```python
from build123d import *

# Parameters (mm, degrees)
F0_W      = 300
F0_H      = 10
F1_DEPTH  = 300
F2_W      = 25
F2_H      = 25
F3_DEPTH  = 10
F4_W      = 20
F4_H      = 10
F5_DEPTH  = 1
F6_W      = 20
F6_H      = 10
F7_DEPTH  = 1
F8_W      = 1
F8_H      = 20
F9_DEPTH  = 200
F10_W     = 300
F10_H     = 10
F11_DEPTH = 300


with BuildPart() as f1:
    # F0 (on Front) → F1 (new body)
    with BuildSketch(Plane.XZ):
        with Locations((102.931539, 34.842865)):
            Rectangle(F0_W, F0_H)
    extrude(amount=F1_DEPTH)

    # F2 (on face) → F3 (join)
    with BuildSketch(Plane(origin=(0, 0, 29.842865), x_dir=(1, 0, 0), z_dir=(0, 0, -1))):
        with Locations((240.431539, 12.5)):
            Rectangle(F2_W, F2_H)
        with Locations((-34.568461, 12.5)):
            Rectangle(F2_W, F2_H)
        with Locations((240.431539, 287.5)):
            Rectangle(F2_W, F2_H)
        with Locations((-34.568461, 287.5)):
            Rectangle(F2_W, F2_H)
    extrude(amount=F3_DEPTH)

    # F4 (on face) → F5 (join)
    with BuildSketch(Plane.YZ.offset(252.931539)):
        with Locations((-45, 34.842865)):
            Rectangle(F4_W, F4_H)
        with Locations((-255, 34.842865)):
            Rectangle(F4_W, F4_H)
    extrude(amount=F5_DEPTH)

    # F6 (on face) → F7 (join)
    with BuildSketch(Plane(origin=(-47.068461, 0, 0), x_dir=(0, -1, 0), z_dir=(-1, 0, 0))):
        with Locations((45, 34.842865)):
            Rectangle(F6_W, F6_H)
        with Locations((255, 34.842865)):
            Rectangle(F6_W, F6_H)
    extrude(amount=F7_DEPTH)

    # F8 (on face) → F9 (join)
    with BuildSketch(Plane.XY.offset(39.842865)):
        with Locations((253.431539, -45)):
            Rectangle(F8_W, F8_H)
        with Locations((253.431539, -255)):
            Rectangle(F8_W, F8_H)
        with Locations((-47.568461, -255)):
            Rectangle(F8_W, F8_H)
        with Locations((-47.568461, -45)):
            Rectangle(F8_W, F8_H)
    extrude(amount=F9_DEPTH)

    # F10 (on face) → F11 (join)
    with BuildSketch(Plane(origin=(252.931539, 0, 0), x_dir=(0, -1, 0), z_dir=(-1, 0, 0))):
        with Locations((150, 234.842865)):
            Rectangle(F10_W, F10_H)
    extrude(amount=F11_DEPTH)


solid = f1.part
```
Check sheet for the modelled part. Datum: model origin and axes. Units: mm. A direction names the side the tool comes from. Give positions to 0.01 mm unless a question says otherwise; leave off trailing zeros. Write each loop counter-clockwise with the first axis right and the second up, starting at its lowest first coordinate (ties: lowest second). Pieces come first, ordered by that corner, then holes. Notation, with made-up numbers: (-22, 65) -> (27, 65) arc R36 ccw to (27, 102) -> close; hole circle Ø6 at (1, 1.5). An arc over 180 degrees is marked (long way). Use CSV: the item, a comma, the result in double quotes. Start each with the question number.
Q1. Scan lines: line 1 along Z through (x, y) = (110, -73); line 2 along X through (y, z) = (-258.5, 58.5). Record each from-to range of solid material in increasing order.
Q2. Cross-section at B-B on y = -61. Enter the section's corners in (x, z).
Q3. Cross-section at C-C on x = 177. Enter the section's corners in (y, z), and give its area (3 significant figures).
Q4. Release check for a two-part mould opening along Y. For faces 6 (the flat face through (105, -148, 239.843)), 7 (the flat face through (240, -25, 25)), 8 (the flat face through (105, 0, 235)) record: +Y half, -Y half, draft (parallel to the pull), parting line (faces both ways), or undercut.
Q5. Tool access check on faces 1 (the flat face through (-47.068, -149, 235)), 2 (the flat face through (-22.068, -12, 25)), 3 (the flat face through (252.932, -255, 134)), 4 (the flat face through (252.932, -17, 235)), 5 (the flat face through (-47.068, -286, 30)). Record the directions out of +Z, -Z, +X, -X, +Y, -Y that give a thin tool (end or side, any length) a straight path to the whole face; none if there is none.
Q6. Depth check by flat-ended pin: P1, Ø10, axis at y = -275, z = 25, coming from the -X side; P2, Ø3, axis at y = -26, z = 235.5, coming from the +X side; P3, Ø1.1, axis at x = 253.5, z = 178, coming from the -Y side. Enter the tip coordinate at first touch or a pass-through.
Q7. Cross-section at A-A on z = 136. Enter the section's corners in (x, y).
Working result:
1,line 1,"z = 29.84 to 39.84, 229.84 to 239.84"
1,line 2,"x = -48.07 to -47.07, 252.93 to 253.93"
2,outline,"(-47.07, 29.84) -> (252.93, 29.84) -> (252.93, 39.84) -> (-47.07, 39.84) -> close; (-47.07, 229.84) -> (252.93, 229.84) -> (252.93, 239.84) -> (-47.07, 239.84) -> close"
3,outline,"(-300, 29.84) -> (0, 29.84) -> (0, 39.84) -> (-300, 39.84) -> close; (-300, 229.84) -> (0, 229.84) -> (0, 239.84) -> (-300, 239.84) -> close"
3,area,"6,000 mm^2"
4,face 6,"draft"
4,face 7,"undercut"
4,face 8,"+Y half"
5,face 1,"+Z, -Z, -X"
5,face 2,"-Z, +Y, -Y"
5,face 3,"+Y, -Y"
5,face 4,"+Z, -Z, +X, +Y"
5,face 5,"+Z, -Z, -X, -Y"
6,P1,"stops at x = -47.07"
6,P2,"stops at x = 252.93"
6,P3,"stops at y = -265"
7,outline,"(-48.07, -265) -> (-47.07, -265) -> (-47.07, -245) -> (-48.07, -245) -> close; (-48.07, -55) -> (-47.07, -55) -> (-47.07, -35) -> (-48.07, -35) -> close; (252.93, -265) -> (253.93, -265) -> (253.93, -245) -> (252.93, -245) -> close; (252.93, -55) -> (253.93, -55) -> (253.93, -35) -> (252.93, -35) -> close"
